Check sheet for the modelled part. Datum: model origin and axes. Units: mm. Face numbers are marked on the shaded views. Round coordinates to 2 decimals unless told otherwise and drop trailing zeros. Order: outer loops, then holes, each group sorted by start corner. A loop starts at its lowest first (then second) coordinate and runs counter-clockwise, first axis right, second up. Notation, with made-up numbers: (26, -25) -> (46, -25) arc R20 cw to (46, 12) -> close; hole circle Ø5 at (37.25, 16.25). An arc over 180 degrees is marked (long way). Answer in a Markdown table with one row per item.
from build123d import *

# Parameters (mm, degrees)
EXTRUDE_1_DEPTH     = 10
EXTRUDE_START       = -10
EXTRUDE_2_DEPTH     = 10
EXTRUDE_4_DEPTH     = 10
SKETCH_3_R          = 2.25
CUT_EXTRUDE_4_DEPTH = 62.923824171
SKETCH_4_R          = 2.25
CUT_EXTRUDE_2_DEPTH = 62.184638595
FILLET_2_R          = 1
EXTRUDE_3_DEPTH     = 10
CUT_EXTRUDE_3_DEPTH = 62.923824171
FILLET_3_R          = 1
FILLET_4_R          = 2


with BuildPart() as part:
    # Эскиз1 → Бобышка-Вытянуть1 (new body)
    with BuildSketch(Plane(origin=(0, 0, 0), x_dir=(1, 0, 0), z_dir=(0, 1, 0))):
        with BuildLine():
            Line((0, 0), (0, 8))
            ThreePointArc((0, 8), (-7.1, 15.1), (0, 22.2))
            Line((0, 22.2), (0, 37.8))
            ThreePointArc((0, 37.8), (-7.1, 44.9), (0, 52))
            Line((0, 52), (0, 60))
            Line((0, 60), (-3, 60))
            Line((-3, 60), (-3, 54.544169223))
            ThreePointArc((-3, 54.544169223), (-10.1, 44.9), (-3, 35.255830777))
            Line((-3, 35.255830777), (-3, 24.744169223))
            ThreePointArc((-3, 24.744169223), (-10.1, 15.1), (-3, 5.455830777))
            Line((-3, 5.455830777), (-3, 0))
            Line((-3, 0), (0, 0))
        make_face()
    extrude(amount=EXTRUDE_1_DEPTH)

    # Эскиз2 → Бобышка-Вытянуть2 (add)
    with BuildSketch(Plane(origin=(0, 10, 0), x_dir=(1, 0, 0), z_dir=(0, 1, 0)).offset(EXTRUDE_START)):
        with BuildLine():
            Line((-3, 60), (-8.049844719, 60))
            Line((-8.049844719, 60), (-8.049844719, 51))
            ThreePointArc((-8.049844719, 51), (-5.802159163, 53.167100402), (-3, 54.544169223))
            Line((-3, 54.544169223), (-3, 60))
        make_face()
        with BuildLine():
            Line((-3, 0), (-3, 5.455830777))
            ThreePointArc((-3, 5.455830777), (-5.802159163, 6.832899598), (-8.049844719, 9))
            Line((-8.049844719, 9), (-8.049844719, 0))
            Line((-8.049844719, 0), (-3, 0))
        make_face()
    extrude(amount=EXTRUDE_2_DEPTH)

    # Эскиз9 → Бобышка-Вытянуть4 (add, through all)
    with BuildSketch(Plane.XZ):
        with BuildLine():
            Line((-5, -25.567091287), (-5, -34.432908713))
            ThreePointArc((-5, -34.432908713), (-11.207890559, -41.909483454), (-9.549844719, -51.484866426))
            Line((-9.549844719, -51.484866426), (-9.549844719, -60))
            Line((-9.549844719, -60), (-8.049844719, -60))
            Line((-8.049844719, -60), (-8.049844719, -51))
            ThreePointArc((-8.049844719, -51), (-9.617405222, -41.81527687), (-3, -35.255830777))
            Line((-3, -35.255830777), (-3, -24.744169223))
            ThreePointArc((-3, -24.744169223), (-9.617405222, -18.18472313), (-8.049844719, -9))
            Line((-8.049844719, -9), (-8.049844719, 0))
            Line((-8.049844719, 0), (-9.549844719, 0))
            Line((-9.549844719, 0), (-9.549844719, -8.515133574))
            ThreePointArc((-9.549844719, -8.515133574), (-11.207890559, -18.090516546), (-5, -25.567091287))
        make_face()
    extrude(amount=-EXTRUDE_4_DEPTH)

    # Эскиз3 → Вырез-Вытянуть4 (cut, through all)
    with BuildSketch(Plane.ZY):
        with Locations(Location((-55.75, 5, 0), (0, 0, 180))):
            Circle(SKETCH_3_R)
        with Locations(Location((-4.25, 5, 0), (0, 0, 180))):
            Circle(SKETCH_3_R)
    extrude(amount=CUT_EXTRUDE_4_DEPTH, mode=Mode.SUBTRACT)

    # Эскиз4 → Вырез-Вытянуть2 (cut, through all)
    with BuildSketch(Plane.ZY.offset(5)):
        with Locations((-30, 5)):
            Circle(SKETCH_4_R)
    extrude(amount=-CUT_EXTRUDE_2_DEPTH, mode=Mode.SUBTRACT)

    # Скругление2
    fillet_2_edges = [part.edges().sort_by_distance(p)[0] for p in [
        (0, 5, -60),
        (0, 5, 0),
    ]]
    fillet(fillet_2_edges, radius=FILLET_2_R)

    # Эскиз5 → Бобышка-Вытянуть3 (add, through all)
    with BuildSketch(Plane.XZ):
        with BuildLine():
            Line((0, -8), (0, -8.1))
            ThreePointArc((0, -8.1), (-7, -15.1), (0, -22.1))
            Line((0, -22.1), (0, -22.2))
            ThreePointArc((0, -22.2), (-7.1, -15.1), (0, -8))
        make_face()
        with BuildLine():
            Line((0, -51.9), (0, -52))
            ThreePointArc((0, -52), (-7.1, -44.9), (0, -37.8))
            Line((0, -37.8), (0, -37.9))
            ThreePointArc((0, -37.9), (-7, -44.9), (0, -51.9))
        make_face()
    extrude(amount=-EXTRUDE_3_DEPTH)

    # Эскиз7 → Вырез-Вытянуть3 (cut, through all)
    with BuildSketch(Plane(origin=(0, 10, 0), x_dir=(1, 0, 0), z_dir=(0, 1, 0))):
        with BuildLine():
            Line((0, 51.9), (0, 53.4))
            ThreePointArc((0, 53.4), (-8.5, 44.9), (0, 36.4))
            Line((0, 36.4), (0, 37.9))
            ThreePointArc((0, 37.9), (-7, 44.9), (0, 51.9))
        make_face()
        with BuildLine():
            Line((0, 22.1), (0, 23.6))
            ThreePointArc((0, 23.6), (-8.5, 15.1), (0, 6.6))
            Line((0, 6.6), (0, 8.1))
            ThreePointArc((0, 8.1), (-7, 15.1), (0, 22.1))
        make_face()
    extrude(amount=-CUT_EXTRUDE_3_DEPTH, mode=Mode.SUBTRACT)

    # Скругление3
    fillet_3_edges = [part.edges().sort_by_distance(p)[0] for p in [
        (-9.549844719, 5, 0),
        (-9.549844719, 5, -60),
    ]]
    fillet(fillet_3_edges, radius=FILLET_3_R)

    # Скругление4
    fillet_4_edges = [part.edges().sort_by_distance(p)[0] for p in [
        (-5, 5, -34.432908713),
        (-5, 5, -25.567091287),
    ]]
    fillet(fillet_4_edges, radius=FILLET_4_R)


solid = part.part
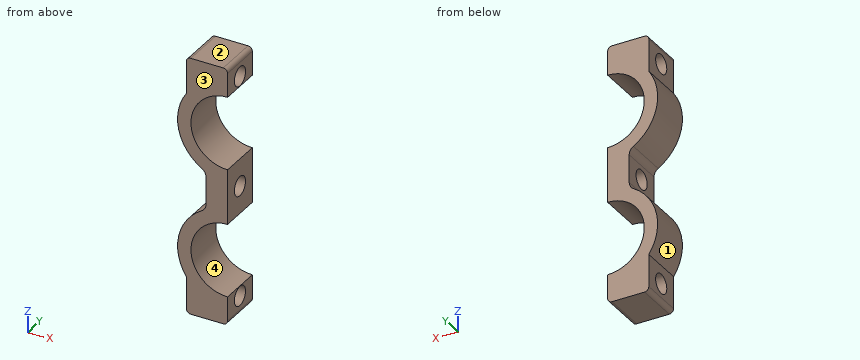
Item 1: Cross-section at D-D (x = -8). Record the boundary of the cut face in (y, z), and give its area (3 significant figures).
Result sheet:
| item | result |
|---|---|
| outline | (0, -60) -> (10, -60) -> (10, -47.77) -> (0, -47.77) -> close; (0, -42.03) -> (10, -42.03) -> (10, -36.5) -> (0, -36.5) -> close; (0, -23.5) -> (10, -23.5) -> (10, -17.97) -> (0, -17.97) -> close; (0, -12.23) -> (10, -12.23) -> (10, 0) -> (0, 0) -> close; hole circle Ø4.5 at (5, -55.75); hole circle Ø4.5 at (5, -4.25) |
| area | 323 mm^2 |
Item 2: Scan lines: line 1 (Y direction, x = -2.3, z = -30); line 2 (Z direction, x = -4.25, y = 3); line 3 (Z direction, x = -4, y = 3). Record each from-to range of solid material in increasing order. Write a range as [from, to].
Result sheet:
| item | result |
|---|---|
| line 1 | y = [0, 2.75], [7.25, 10] |
| line 2 | z = [-60, -56.78], [-54.72, -52.26], [-37.54, -31.03], [-28.97, -22.46], [-7.74, -5.28], [-3.22, 0] |
| line 3 | z = [-60, -56.78], [-54.72, -52.4], [-37.4, -31.03], [-28.97, -22.6], [-7.6, -5.28], [-3.22, 0] |
Item 3: Mould release check, pull along Z, two halves, no side actions. Record for the marked faces 1, 2, 3 and 4: pulls with the +Z half, pulls with the -Z half, needs draft (parallel to the pull), parting line crosses it, or undercut.
Result sheet:
| item | result |
|---|---|
| face 1 | undercut |
| face 2 | pulls with the +Z half |
| face 3 | needs draft |
| face 4 | undercut |
Item 4: Cross-section at C-C (y = 5). State how many separate pieces and enclosed holes the cut face has, and give its area (3 significant figures).
Result sheet:
| item | result |
|---|---|
| separate pieces | 4 |
| enclosed holes | 0 |
| area | 219 mm^2 |
Item 5: Depth check by flat-ended pin: P1, Ø6, axis at y = 5, z = -55.75, coming from the -X side; P2, Ø1, axis at y = 1.5, z = -31.5, coming from the -X side; P3, Ø6, axis at y = 9, z = -6.5, coming from the -X side. Enter the tip coordinate at first touch or a pass-through.
Result sheet:
| item | result |
|---|---|
| P1 | stops at x = -9.55 |
| P2 | stops at x = -5 |
| P3 | stops at x = -10.16 |
Item 6: Cross-section at B-B (z = -30). Record the boundary of the cut face in (x, y).
Result sheet:
| item | result |
|---|---|
| outline | (-5, 0) -> (0, 0) -> (0, 2.75) -> (-5, 2.75) -> close; (-5, 7.25) -> (0, 7.25) -> (0, 10) -> (-5, 10) -> close |
Item 7: Cross-section at A-A (x = -4.25). Record the boundary of the cut face in (y, z).
Result sheet:
| item | result |
|---|---|
| outline | (0, -60) -> (10, -60) -> (10, -52.26) -> (0, -52.26) -> close; (0, -37.54) -> (10, -37.54) -> (10, -22.46) -> (0, -22.46) -> close; (0, -7.74) -> (10, -7.74) -> (10, 0) -> (0, 0) -> close; hole circle Ø4.5 at (5, -55.75); hole circle Ø4.5 at (5, -30); hole circle Ø4.5 at (5, -4.25) |
